Check sheet for the modelled part. Datum: model origin and axes. Units: mm. Give positions to 0.01 mm unless a question says otherwise; leave off trailing zeros. Write each loop counter-clockwise with the first axis right and the second up, starting at its lowest first coordinate (ties: lowest second). Pieces come first, ordered by that corner, then holes. Notation, with made-up numbers: (37.25, -27.75) -> (63.25, -27.75) arc R22 ccw to (63.25, -10.75) -> close; hole circle Ø7 at (59, 15). An arc over 180 degrees is marked (long way). Use a Markdown table: item, result. Add a question column.
1. Gauge pin test, flat end, axial feed: P1, Ø0.8, axis at x = 8.06, z = -6.16, coming from the +Y side. Record the tip position at first contact, or that the pin passes through.
2. Cross-section at A-A (x = -1.34). Enter the section's corners in (y, z), then the cut area to 3 significant figures.
3. Cross-section at B-B (z = -3.81). Count the separate pieces of the cut face and the enclosed holes in it, then the cut area to 3 significant figures.
4. Release check for a two-part mould opening along X. For faces 1 (the flat face through (-12.5, 0.5, 0.2)), 2 (the cylindrical face through (-4.39, 0.49, -1.49)), 3 (the flat face through (12.5, 0.5, 0.2)) record: released by +X, released by -X, zero draft, split by the parting line, or undercut.
5. Scan lines: probe 1 along Z at (x, y) = (5.71, 0.2); probe 2 along Z at (x, y) = (8.25, 0.3). Record each from-to range of solid material in increasing order. Write a range as [from, to].
from build123d import *

# Parameters (mm, degrees)
SKETCH1_W           = 25
SKETCH1_H           = 25
SKETCH1_R           = 0.7
BOSS_EXTRUDE1_DEPTH = 1


with BuildPart() as part:
    # Sketch1 → Boss-Extrude1 (new body)
    with BuildSketch(Plane(origin=(0, 0, 0), x_dir=(1, 0, 0), z_dir=(0, 1, 0))):
        Rectangle(SKETCH1_W, SKETCH1_H)
        with Locations((-8.39, 8.51)):
            Circle(SKETCH1_R, mode=Mode.SUBTRACT)
        with Locations((-6.04, 8.51)):
            Circle(SKETCH1_R, mode=Mode.SUBTRACT)
        with Locations((-3.69, 8.51)):
            Circle(SKETCH1_R, mode=Mode.SUBTRACT)
        with Locations((-1.34, 8.51)):
            Circle(SKETCH1_R, mode=Mode.SUBTRACT)
        with Locations((1.01, 8.51)):
            Circle(SKETCH1_R, mode=Mode.SUBTRACT)
        with Locations((3.36, 8.51)):
            Circle(SKETCH1_R, mode=Mode.SUBTRACT)
        with Locations((5.71, 8.51)):
            Circle(SKETCH1_R, mode=Mode.SUBTRACT)
        with Locations((8.06, 8.51)):
            Circle(SKETCH1_R, mode=Mode.SUBTRACT)
        with Locations((-6.04, 6.16)):
            Circle(SKETCH1_R, mode=Mode.SUBTRACT)
        with Locations((-3.69, 6.16)):
            Circle(SKETCH1_R, mode=Mode.SUBTRACT)
        with Locations((-1.34, 6.16)):
            Circle(SKETCH1_R, mode=Mode.SUBTRACT)
        with Locations((1.01, 6.16)):
            Circle(SKETCH1_R, mode=Mode.SUBTRACT)
        with Locations((3.36, 6.16)):
            Circle(SKETCH1_R, mode=Mode.SUBTRACT)
        with Locations((5.71, 6.16)):
            Circle(SKETCH1_R, mode=Mode.SUBTRACT)
        with Locations((8.06, 6.16)):
            Circle(SKETCH1_R, mode=Mode.SUBTRACT)
        with Locations((-6.04, 3.81)):
            Circle(SKETCH1_R, mode=Mode.SUBTRACT)
        with Locations((-3.69, 3.81)):
            Circle(SKETCH1_R, mode=Mode.SUBTRACT)
        with Locations((-1.34, 3.81)):
            Circle(SKETCH1_R, mode=Mode.SUBTRACT)
        with Locations((1.01, 3.81)):
            Circle(SKETCH1_R, mode=Mode.SUBTRACT)
        with Locations((3.36, 3.81)):
            Circle(SKETCH1_R, mode=Mode.SUBTRACT)
        with Locations((5.71, 3.81)):
            Circle(SKETCH1_R, mode=Mode.SUBTRACT)
        with Locations((8.06, 3.81)):
            Circle(SKETCH1_R, mode=Mode.SUBTRACT)
        with Locations((-6.04, 1.46)):
            Circle(SKETCH1_R, mode=Mode.SUBTRACT)
        with Locations((-3.69, 1.46)):
            Circle(SKETCH1_R, mode=Mode.SUBTRACT)
        with Locations((-1.34, 1.46)):
            Circle(SKETCH1_R, mode=Mode.SUBTRACT)
        with Locations((1.01, 1.46)):
            Circle(SKETCH1_R, mode=Mode.SUBTRACT)
        with Locations((3.36, 1.46)):
            Circle(SKETCH1_R, mode=Mode.SUBTRACT)
        with Locations((5.71, 1.46)):
            Circle(SKETCH1_R, mode=Mode.SUBTRACT)
        with Locations((8.06, 1.46)):
            Circle(SKETCH1_R, mode=Mode.SUBTRACT)
        with Locations((-8.39, 6.16)):
            Circle(SKETCH1_R, mode=Mode.SUBTRACT)
        with Locations((-8.39, 3.81)):
            Circle(SKETCH1_R, mode=Mode.SUBTRACT)
        with Locations((-8.39, 1.46)):
            Circle(SKETCH1_R, mode=Mode.SUBTRACT)
    extrude(amount=BOSS_EXTRUDE1_DEPTH)


solid = part.part
Worked answers:
| question | item | result |
|---|---|---|
| 1 | P1 | passes through |
| 2 | outline | (0, -12.5) -> (1, -12.5) -> (1, -9.21) -> (0, -9.21) -> close; (0, -7.81) -> (1, -7.81) -> (1, -6.86) -> (0, -6.86) -> close; (0, -5.46) -> (1, -5.46) -> (1, -4.51) -> (0, -4.51) -> close; (0, -3.11) -> (1, -3.11) -> (1, -2.16) -> (0, -2.16) -> close; (0, -0.76) -> (1, -0.76) -> (1, 12.5) -> (0, 12.5) -> close |
| 2 | area | 19.4 mm² |
| 3 | separate pieces | 9 |
| 3 | enclosed holes | 0 |
| 3 | area | 13.8 mm² |
| 4 | face 1 | released by -X |
| 4 | face 2 | undercut |
| 4 | face 3 | released by +X |
| 5 | probe 1 | z = [-12.5, -9.21], [-7.81, -6.86], [-5.46, -4.51], [-3.11, -2.16], [-0.76, 12.5] |
| 5 | probe 2 | z = [-12.5, -9.18], [-7.84, -6.83], [-5.49, -4.48], [-3.14, -2.13], [-0.79, 12.5] |
